The listing builds one solid part. Answer for the finished solid, in the listing's coordinates (mm). A direction names the side the tool comes from. Coordinates: 2 decimals unless noted, no trailing zeros. Order: outer loops, then holes, each group sorted by start corner. A loop starts at its lowest first (then second) coordinate and runs counter-clockwise, first axis right, second up. Notation, with made-up numbers: (21.25, -24) -> (27.25, -24) arc R8 ccw to (27.25, -16) -> close; hole circle Ø6 at (-34.5, 27). An arc over 180 degrees is marked (long way). Return JSON: item names as keys, results as strings.
```python
from build123d import *

# Parameters (mm, degrees)
SKETCH_1_R          = 1
EXTRUDE_1_DEPTH     = 25.5
SKETCH_2_W          = 8
SKETCH_2_H          = 4
CUT_EXTRUDE_2_DEPTH = 3
CUT_EXTRUDE_3_DEPTH = 8
CUT_EXTRUDE_START   = -9
CUT_EXTRUDE_4_DEPTH = 12
EXTRUDE_2_DEPTH     = 0.5


with BuildPart() as part:
    # 草图1 → 凸台-拉伸1 (new body)
    with BuildSketch(Plane.XY):
        with BuildLine():
            Line((0, 2), (43, 2))
            Line((43, 2), (43, -6))
            Line((43, -6), (41, -6))
            Line((41, -6), (41, -2))
            Line((41, -2), (0, -2))
            ThreePointArc((0, -2), (-2, 0), (0, 2))
        make_face()
        Circle(SKETCH_1_R, mode=Mode.SUBTRACT)
    extrude(amount=EXTRUDE_1_DEPTH)

    # 草图2 → 切除-拉伸2 (cut)
    with BuildSketch(Plane.XY.offset(25.5)):
        Rectangle(SKETCH_2_W, SKETCH_2_H)
    extrude(amount=-CUT_EXTRUDE_2_DEPTH, mode=Mode.SUBTRACT)

    # 草图3 → 切除-拉伸3 (cut)
    with BuildSketch(Plane(origin=(0, 0, 0), x_dir=(-1, 0, 0), z_dir=(0, 0, -1))):
        with BuildLine():
            Line((0, 2), (-4, 2))
            Line((-4, 2), (-4, -2))
            Line((-4, -2), (0, -2))
            ThreePointArc((0, -2), (2, 0), (0, 2))
        make_face()
    extrude(amount=-CUT_EXTRUDE_3_DEPTH, mode=Mode.SUBTRACT)

    # 草图3<2> → 切除-拉伸4 (cut)
    with BuildSketch(Plane(origin=(0, 0, 0), x_dir=(-1, 0, 0), z_dir=(0, 0, -1)).offset(CUT_EXTRUDE_START)):
        with BuildLine():
            ThreePointArc((0, -2), (2, 0), (0, 2))
            Line((0, 2), (-4, 2))
            Line((-4, 2), (-4, -2))
            Line((-4, -2), (0, -2))
        make_face()
    extrude(amount=-CUT_EXTRUDE_4_DEPTH, mode=Mode.SUBTRACT)

    # 草图4 → 凸台-拉伸2 (add)
    with BuildSketch(Plane.ZY.offset(-41)):
        Polygon((13.75, -5.068409561), (11.75, -5.068409561), (11.75, -6), (12.75, -6), (13.75, -6), align=None)
    extrude(amount=EXTRUDE_2_DEPTH)


solid = part.part
```
Item 1: The part is cut by section A-A on y = 0. Determine the outline of the cut face in (x, z).
Answer list:
{"outline": "(-2, 8) -> (-1, 8) -> (-1, 9) -> (-2, 9) -> close; (-2, 21) -> (-1, 21) -> (-1, 22.5) -> (-2, 22.5) -> close; (1, 8) -> (4, 8) -> (4, 0) -> (43, 0) -> (43, 25.5) -> (4, 25.5) -> (4, 22.5) -> (1, 22.5) -> (1, 21) -> (4, 21) -> (4, 9) -> (1, 9) -> close"}
Item 2: Determine the mould class of faces 6 (the flat face through (2, 0, 8)), 7 (the cylindrical face through (0, -1, 22)), 8 (the flat face through (2, 0, 21)) for opening direction Z: pulls with the +Z half, pulls with the -Z half, needs draft (parallel to the pull), parting line crosses it, or undercut.
Answer list:
{"face 6": "pulls with the -Z half", "face 7": "needs draft", "face 8": "undercut"}
Item 3: The part is cut by section D-D on x = 24.5. Determine the outline of the cut face in (y, z), plus the area to 3 significant figures.
Answer list:
{"outline": "(-2, 0) -> (2, 0) -> (2, 25.5) -> (-2, 25.5) -> close", "area": "102 mm2"}
Item 4: The part is cut by section B-B on z = 8.5. Determine the outline of the cut face in (x, y), plus the area to 3 significant figures.
Answer list:
{"outline": "(0, -2) -> (41, -2) -> (41, -6) -> (43, -6) -> (43, 2) -> (0, 2) arc R2 ccw to start; hole circle Ø2 at (0, 0)", "area": "183 mm2"}
Item 5: The part is cut by section C-C on z = 12.5. Determine the outline of the cut face in (x, y), plus the area to 3 significant figures.
Answer list:
{"outline": "(4, -2) -> (41, -2) -> (41, -5.07) -> (40.5, -5.07) -> (40.5, -6) -> (43, -6) -> (43, 2) -> (4, 2) -> close", "area": "164 mm2"}
Item 6: Find the intervals of material crossed by probe 1 along X at (y, z) = (0, 22.05); probe 2 along Y at (x, z) = (0, 8.5); probe 3 along Y at (x, z) = (7, 8.25), in increasing order.
Answer list:
{"probe 1": "-2 to -1, 1 to 43", "probe 2": "-2 to -1, 1 to 2", "probe 3": "-2 to 2"}
Item 7: Flat-ended cylindrical pins translate along their axes: pin 1 (2 mm diameter, centred on x = 2, y = 0.5, fed in from +Z); pin 2 (5 mm diameter, centred on x = 22.5, z = 11.5, fed in from -Y); pin 3 (4.5 mm diameter, centred on y = 1, z = 2.5, fed in from -X); pin 4 (1.8 mm diameter, centred on x = 0, y = 0, fed in from -Z). Find the tip coordinate at first contact, or state that the pin passes through.
Answer list:
{"pin 1": "z = 22.5", "pin 2": "y = -2", "pin 3": "x = 4", "pin 4": "through"}
Item 8: Which of the six approach directions +Z, -Z, +X, -X, +Y, -Y give full straight-line access (tool end or side, diameter ignored) to faces 1 (the flat face through (24, 0, 25.5)), 2 (the flat face through (4, 0, 15)), 3 (the flat face through (4, 0, 4)), 4 (the flat face through (40.5, -5.5, 12.7)), 5 (the flat face through (4, 0, 24))?
Answer list:
{"face 1": "+Z, +X, -X, +Y, -Y", "face 2": "-X, +Y, -Y", "face 3": "-Z, -X, +Y, -Y", "face 4": "+Z, -Z, -X, -Y", "face 5": "+Z, -X, +Y, -Y"}
